```python
from build123d import *

# Parameters (mm, degrees)
F0_R     = 1.1811
F0_R_2   = 1.5875
F1_DEPTH = 1.5875
F2_SIZE  = 0.508


with BuildPart() as f1:
    # F0 (on Front) → F1 (new body, symmetric)
    with BuildSketch(Plane.XZ):
        with BuildLine():
            Line((5.750813, 4.094138), (-6.573008, 4.094138))
            ThreePointArc((-6.573008, 4.094138), (-4.49461, -3.713278), (3.584436, -3.780322))
            Line((3.584436, -3.780322), (5.750813, 4.094138))
        make_face()
        with Locations((-0.411098, -3.459583)):
            Circle(F0_R, mode=Mode.SUBTRACT)
        with Locations((-0.411098, 1.554138)):
            Circle(F0_R_2, mode=Mode.SUBTRACT)
    extrude(amount=F1_DEPTH, both=True)

    # F2
    f2_edges = [f1.edges().sort_by_distance(p)[0] for p in [
        (5.750813, 0, 4.094138),
    ]]
    chamfer(f2_edges, length=F2_SIZE)


solid = f1.part
```
Geometry check sheet. Reference: the model listing, model coordinates, mm. Give positions to 0.01 mm unless a question says otherwise; leave off trailing zeros. Write each loop counter-clockwise with the first axis right and the second up, starting at its lowest first coordinate (ties: lowest second). Pieces come first, ordered by that corner, then holes. Notation, with made-up numbers: (83, 74) - (138, 74) arc R16 cw to (138, 83) - close; hole circle Ø4 at (-20.5, 58). An arc over 180 degrees is marked (long way). Use a Markdown table: item, result.
Q1. Go/stop test with flat-tipped pins: P1, Ø1.9, axis at x = -0.41, z = 1.55, coming from the +Y side; P2, Ø2.5, axis at x = -0.41, z = -3.46, coming from the -Y side. Record where each tip stops, or that it passes through.
Computed:
| item | result |
|---|---|
| P1 | passes through |
| P2 | stops at y = -1.59 |
Q2. Section check D-D, the plane z = 0.25. Enter the section's corners in (x, y).
Computed:
| item | result |
|---|---|
| outline | (-6.95, -1.59) - (-1.32, -1.59) - (-1.32, 1.59) - (-6.95, 1.59) - close; (0.49, -1.59) - (4.69, -1.59) - (4.69, 1.59) - (0.49, 1.59) - close |
Q3. Draft check along X on faces 1 (the face through (-1.58, 0.02, 2.63)), 2 (the face through (4.586, -0.022, -0.14)), 3 (the face through (-0.8, 1.588, -0.4)), 4 (the face through (-1.28, 0.02, -2.66)). Enter one of: pulls with the +X half, pulls with the -X half, needs draft (parallel to the pull), parting line crosses it, or undercut.
Computed:
| item | result |
|---|---|
| face 1 | undercut |
| face 2 | pulls with the +X half |
| face 3 | needs draft |
| face 4 | undercut |
Q4. Section check B-B, the plane x = -0.75. Enter the section's corners in (y, z), then the cut area to 3 significant figures.
Computed:
| item | result |
|---|---|
| outline | (-1.59, -5.1) - (1.59, -5.1) - (1.59, -4.59) - (-1.59, -4.59) - close; (-1.59, -2.33) - (1.59, -2.33) - (1.59, 0) - (-1.59, 0) - close; (-1.59, 3.11) - (1.59, 3.11) - (1.59, 4.09) - (-1.59, 4.09) - close |
| area | 12.2 mm² |
Q5. Section check C-C, the plane y = 0.95. Enter the section's corners in (x, z) (1 decimal).
Computed:
| item | result |
|---|---|
| outline | (-6.6, 4.1) arc R6.7 ccw to (3.6, -3.8) - (5.6, 3.6) - (5.2, 4.1) - close; hole circle Ø3.2 at (-0.4, 1.6); hole circle Ø2.4 at (-0.4, -3.5) |
Q6. Thickness scan on L1, parallel to X at y = 0.3, z = 2.25; L2, parallel to X at y = 1.25, z = -4; L3, parallel to Z at x = -1.75, y = -0.85. Record the ranges inside material, lowest first. Write a range as [from, to].
Computed:
| item | result |
|---|---|
| L1 | x = [-7.04, -1.84], [1.02, 5.24] |
| L2 | x = [-4.1, -1.46], [0.64, 3.27] |
| L3 | z = [-4.97, 0.7], [2.41, 4.09] |
Q7. Section check A-A, the plane z = 2.5. Enter the section's corners in (x, y).
Computed:
| item | result |
|---|---|
| outline | (-7.01, -1.59) - (-1.69, -1.59) - (-1.69, 1.59) - (-7.01, 1.59) - close; (0.86, -1.59) - (5.31, -1.59) - (5.31, 1.59) - (0.86, 1.59) - close |
